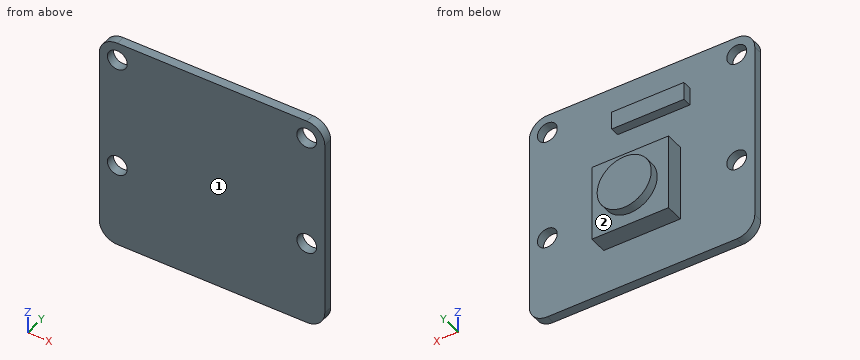
Autodesk Inventor part; units mm, degrees
ref_plane "YZ Plane" through (0, 0, 0) normal (1, 0, 0) x (0, 1, 0)
ref_plane "XZ Plane" through (0, 0, 0) normal (0, 1, 0) x (-1, 0, 0)
ref_plane "XY Plane" through (0, 0, 0) normal (0, 0, 1) x (1, 0, 0)
sketch "Sketch1" plane through (0, 0, 0) normal (0, 1, 0) x (-1, 0, 0)
  line L0 (0, 0) -> (25, 0)
  line L1 (25, 0) -> (25, -23.862)
  line L2 (25, -23.862) -> (0, -23.862)
  line L3 (0, -23.862) -> (0, 0)
  line L4 (0, 0) -> (0, -2)
  line L5 (0, -2) -> (2, -2)
  line L6 (25, 0) -> (25, -2)
  line L7 (25, -2) -> (23, -2)
  circle A0 centre (2, -2) radius 1.1
  circle A1 centre (23, -2) radius 1.1
  line L8 (0, -2) -> (0, -14.5)
  line L9 (0, -14.5) -> (2, -14.5)
  line L10 (23, -2) -> (23, -14.5)
  circle A2 centre (23, -14.5) radius 1.1
  circle A3 centre (2, -14.5) radius 1.1
  dimension "d0" = 25
  dimension "d1" = 23.862
  dimension "d2" = 2
  dimension "d3" = 2
  dimension "d4" = 2
  dimension "d5" = 2
  dimension "d6" = 2.2
  dimension "d7" = 2.2
  dimension "d8" = 12.5
  dimension "d9" = 2
  dimension "d10" = 12.5
  dimension "d11" = 2.2
  dimension "d12" = 2.2
extrude "Extrusion1" add sketch "Sketch1" along normal blind 1
fillet "Fillet1" radius 2 4 edges at (0, 0.5, 0) (0, 0.5, -23.862) (-25, 0.5, -23.862) (-25, 0.5, 0)
sketch "Sketch2" plane through (0, 1, 0) normal (0, 1, 0) x (1, 0, 0)
  arc A0 (-25, 2) -> (-23, 0) centre (-23, 2) ccw
  line L0 (-23, 0) -> (-2, 0)
  arc A1 (-2, 0) -> (0, 2) centre (-2, 2) ccw
  line L1 (0, 2) -> (0, 21.862)
  arc A2 (0, 21.862) -> (-2, 23.862) centre (-2, 21.862) ccw
  line L2 (-2, 23.862) -> (-23, 23.862)
  arc A3 (-23, 23.862) -> (-25, 21.862) centre (-23, 21.862) ccw
  line L3 (-25, 21.862) -> (-25, 2)
  circle A4 centre (-23, 14.5) radius 1.1
  circle A5 centre (-23, 2) radius 1.1
  circle A6 centre (-2, 14.5) radius 1.1
  circle A7 centre (-2, 2) radius 1.1
  circle A8 centre (-23, 14.5) radius 1.1
  circle A9 centre (-2, 14.5) radius 1.1
  line L4 (-23, 14.5) -> (-2, 14.5)
  line L5 (-12.5, 14.5) -> (-16.75, 14.5)
  line L6 (-16.75, 14.5) -> (-16.75, 10.25)
  line L7 (-16.75, 10.25) -> (-8.25, 10.25)
  line L8 (-8.25, 10.25) -> (-8.25, 18.75)
  line L9 (-8.25, 18.75) -> (-16.75, 18.75)
  line L10 (-16.75, 18.75) -> (-16.75, 10.25)
  point P0 (0, 0)
  dimension "d16" = 4.25
  dimension "d17" = 4.25
  dimension "d18" = 8.5
  dimension "d19" = 8.5
extrude "Extrusion2" add sketch "Sketch2" along normal blind 2 contours L10 L9 L8 L4 | L4 L8 L7 L6
sketch "Sketch3" plane through (0, 3, 0) normal (0, 1, 0) x (1, 0, 0)
  line L0 (-16.75, 18.75) -> (-16.75, 10.25)
  line L1 (-16.75, 10.25) -> (-8.25, 10.25)
  line L2 (-8.25, 10.25) -> (-8.25, 18.75)
  line L3 (-8.25, 18.75) -> (-16.75, 18.75)
  circle A0 centre (-12.5, 14.5) radius 3
  point P0 (0, 0)
  dimension "d22" = 6
extrude "Extrusion3" add sketch "Sketch3" along normal blind 1 contours A0
sketch "Sketch4" plane through (0, 1, 0) normal (0, 1, 0) x (1, 0, 0)
  line L0 (-16.75, 18.75) -> (-8.25, 18.75)
  line L1 (-8.25, 18.75) -> (-8.25, 10.25)
  line L2 (-8.25, 10.25) -> (-16.75, 10.25)
  line L3 (-16.75, 10.25) -> (-16.75, 18.75)
  arc A0 (-25, 2) -> (-23, 0) centre (-23, 2) ccw
  line L4 (-23, 0) -> (-2, 0)
  arc A1 (-2, 0) -> (0, 2) centre (-2, 2) ccw
  line L5 (0, 2) -> (0, 21.862)
  arc A2 (0, 21.862) -> (-2, 23.862) centre (-2, 21.862) ccw
  line L6 (-2, 23.862) -> (-23, 23.862)
  arc A3 (-23, 23.862) -> (-25, 21.862) centre (-23, 21.862) ccw
  line L7 (-25, 21.862) -> (-25, 2)
  circle A4 centre (-23, 14.5) radius 1.1
  circle A5 centre (-23, 2) radius 1.1
  circle A6 centre (-2, 14.5) radius 1.1
  circle A7 centre (-2, 2) radius 1.1
  line L8 (0, 0) -> (-13.8, 0)
  line L9 (-23, 0) -> (-2, 0)
  line L10 (-13.8, 0) -> (-13.8, 4.7)
  line L11 (-13.8, 4.7) -> (-9.8, 4.7)
  line L12 (-9.8, 4.7) -> (-9.8, 5.7)
  line L13 (-9.8, 5.7) -> (-17.8, 5.7)
  line L14 (-17.8, 5.7) -> (-17.8, 3.7)
  line L15 (-17.8, 3.7) -> (-9.8, 3.7)
  line L16 (-9.8, 3.7) -> (-9.8, 5.7)
  dimension "d25" = 13.8
  dimension "d26" = 4.7
  dimension "d27" = 4
  dimension "d28" = 1
  dimension "d29" = 8
  dimension "d30" = 2
extrude "Extrusion4" add sketch "Sketch4" along normal blind 1 contours L15 L14 L13 L12 L11 L10 | L10 L11 L16 L15
properties part number "rpiCam"
Verification items for the finished model (mm, model axes). Face numbers are marked on the shaded views. A direction names the side the tool comes from. Give positions to 0.01 mm unless a question says otherwise; leave off trailing zeros. Order: outer loops, then holes, each group sorted by start corner. A loop starts at its lowest first (then second) coordinate and runs counter-clockwise, first axis right, second up. Notation, with made-up numbers: M -25.75,54.5 L 16.25,54.5 A23 ccw 16.25,67.5 Z; hole C 3.25,-12 d11. An arc over 180 degrees is marked long. Return JSON: item names as keys, results as strings. Group by question number.
1) Go/stop test with flat-tipped pins: pin 1 Ø1 at (y, z) = (2.5, -15.5) entering from +X; pin 2 Ø0.8 at (y, z) = (1.5, -5) entering from +X; pin 3 Ø1.6 at (y, z) = (2, -12.5) entering from -X; pin 4 Ø2 at (x, z) = (-2, -14.5) entering from -Y. Record where each tip stops, or that it passes through.
2) Section check D-D on x = -22.25. Record the cut outline in (y, z).
3) Access from +Z, -Z, +X, -X, +Y, -Y to the whole of each face (thin tool, end or side, straight path). Record for the marked faces 1 and 2.
4) Scan lines: line 1 (Z direction, x = -2, y = 0.5); line 2 (X direction, y = 0.5, z = -14.5); line 3 (Z direction, x = -10.5, y = 1.8). Record each from-to range of solid material in increasing order.
5) Section check A-A on z = -14.5. Record the cut outline in (x, y).
6) Section check B-B on y = 1.3. Record the cut outline in (x, z).
7) Section check C-C on x = -12.5. Record the cut outline in (y, z), and give its area (3 significant figures).
Answer block:
{
 "1": {"pin 1": "stops at x = -8.25", "pin 2": "stops at x = -9.8", "pin 3": "stops at x = -16.75", "pin 4": "passes through"},
 "2": {"outline": "M 0,-23.86 L 1,-23.86 L 1,-15.3 L 0,-15.3 Z; M 0,-13.7 L 1,-13.7 L 1,-2.8 L 0,-2.8 Z; M 0,-1.2 L 1,-1.2 L 1,0 L 0,0 Z"},
 "3": {"face 1": "+Z, -Z, +X, -X, -Y", "face 2": "+Y"},
 "4": {"line 1": "z = -23.86 to -15.6, -13.4 to -3.1, -0.9 to 0", "line 2": "x = -25 to -24.1, -21.9 to -3.1, -0.9 to 0", "line 3": "z = -18.75 to -10.25, -5.7 to -3.7"},
 "5": {"outline": "M -25,0 L -24.1,0 L -24.1,1 L -25,1 Z; M -21.9,0 L -3.1,0 L -3.1,1 L -8.25,1 L -8.25,3 L -9.5,3 L -9.5,4 L -15.5,4 L -15.5,3 L -16.75,3 L -16.75,1 L -21.9,1 Z; M -0.9,0 L 0,0 L 0,1 L -0.9,1 Z"},
 "6": {"outline": "M -17.8,-5.7 L -9.8,-5.7 L -9.8,-3.7 L -17.8,-3.7 Z; M -16.75,-18.75 L -8.25,-18.75 L -8.25,-10.25 L -16.75,-10.25 Z"},
 "7": {"outline": "M 0,-23.86 L 1,-23.86 L 1,-18.75 L 3,-18.75 L 3,-17.5 L 4,-17.5 L 4,-11.5 L 3,-11.5 L 3,-10.25 L 1,-10.25 L 1,-5.7 L 2,-5.7 L 2,-3.7 L 1,-3.7 L 1,0 L 0,0 Z", "area": "48.9 mm^2"}
}
